```python
from build123d import *

# Parameters (mm, degrees)
F0_W     = 467.36
F0_H     = 76.2
F0_R     = 8.382
F1_DEPTH = 1.5875


with BuildPart() as f1:
    # F0 (on Top) → F1 (new body)
    with BuildSketch(Plane.XY):
        with Locations((-233.68, 38.1)):
            Rectangle(F0_W, F0_H)
        with Locations((-441.96, 38.1)):
            Circle(F0_R, mode=Mode.SUBTRACT)
        with Locations((-416.56, 38.1)):
            Circle(F0_R, mode=Mode.SUBTRACT)
        with Locations((-386.08, 38.1)):
            Circle(F0_R, mode=Mode.SUBTRACT)
        with Locations((-360.68, 38.1)):
            Circle(F0_R, mode=Mode.SUBTRACT)
        with Locations((-330.2, 38.1)):
            Circle(F0_R, mode=Mode.SUBTRACT)
        with Locations((-304.8, 38.1)):
            Circle(F0_R, mode=Mode.SUBTRACT)
        with Locations((-274.32, 38.1)):
            Circle(F0_R, mode=Mode.SUBTRACT)
        with Locations((-248.92, 38.1)):
            Circle(F0_R, mode=Mode.SUBTRACT)
        with Locations((-218.44, 38.1)):
            Circle(F0_R, mode=Mode.SUBTRACT)
        with Locations((-193.04, 38.1)):
            Circle(F0_R, mode=Mode.SUBTRACT)
        with Locations((-162.56, 38.1)):
            Circle(F0_R, mode=Mode.SUBTRACT)
        with Locations((-137.16, 38.1)):
            Circle(F0_R, mode=Mode.SUBTRACT)
        with Locations((-106.68, 38.1)):
            Circle(F0_R, mode=Mode.SUBTRACT)
        with Locations((-81.28, 38.1)):
            Circle(F0_R, mode=Mode.SUBTRACT)
        with Locations((-50.8, 38.1)):
            Circle(F0_R, mode=Mode.SUBTRACT)
        with Locations((-25.4, 38.1)):
            Circle(F0_R, mode=Mode.SUBTRACT)
    extrude(amount=F1_DEPTH)


solid = f1.part
```
CAD build for the part. Positions are in the model's coordinates, mm. Round coordinates to 2 decimals unless told otherwise and drop trailing zeros. Write each loop counter-clockwise with the first axis right and the second up, starting at its lowest first coordinate (ties: lowest second). Pieces come first, ordered by that corner, then holes. Notation, with made-up numbers: (-36.75, -6) -> (-14.75, -6) arc R29 cw to (-14.75, 26) -> close; hole circle Ø6 at (-35.5, -35.5). An arc over 180 degrees is marked (long way). Answer in a Markdown table with one row per item. Add a question column.
Item 1: Saw through at B-B, the plane z = 0.6. Count the separate pieces of the cut face and the enclosed holes in it, then the cut area to 3 significant figures.
Item 2: Saw through at C-C, the plane x = -247.5. Write the cut outline in (y, z), then the cut area to 3 significant figures.
Item 3: Mould opens along Y. For faces 1 (the face through (-237, 39, 1.588)), 2 (the face through (-408.817, 34.89, 0.783)) say: pulls with the +Y half, pulls with the -Y half, needs draft (parallel to the pull), parting line crosses it, or undercut.
Item 4: Saw through at A-A, the plane x = -25.4. Write the cut outline in (y, z).
Item 5: Drill centre lines: line 1 (Y direction, x = -441.96, z = 1.25); line 2 (Y direction, x = -136, z = 1.2). Where is each one in solid material? Low to high. Write a range as from..to.
Findings below:
| question | item | result |
|---|---|---|
| 1 | separate pieces | 1 |
| 1 | enclosed holes | 16 |
| 1 | area | 32,100 mm^2 |
| 2 | outline | (0, 0) -> (29.84, 0) -> (29.84, 1.59) -> (0, 1.59) -> close; (46.36, 0) -> (76.2, 0) -> (76.2, 1.59) -> (46.36, 1.59) -> close |
| 2 | area | 94.7 mm^2 |
| 3 | face 1 | needs draft |
| 3 | face 2 | undercut |
| 4 | outline | (0, 0) -> (29.72, 0) -> (29.72, 1.59) -> (0, 1.59) -> close; (46.48, 0) -> (76.2, 0) -> (76.2, 1.59) -> (46.48, 1.59) -> close |
| 5 | line 1 | y = 0..29.72, 46.48..76.2 |
| 5 | line 2 | y = 0..29.8, 46.4..76.2 |
